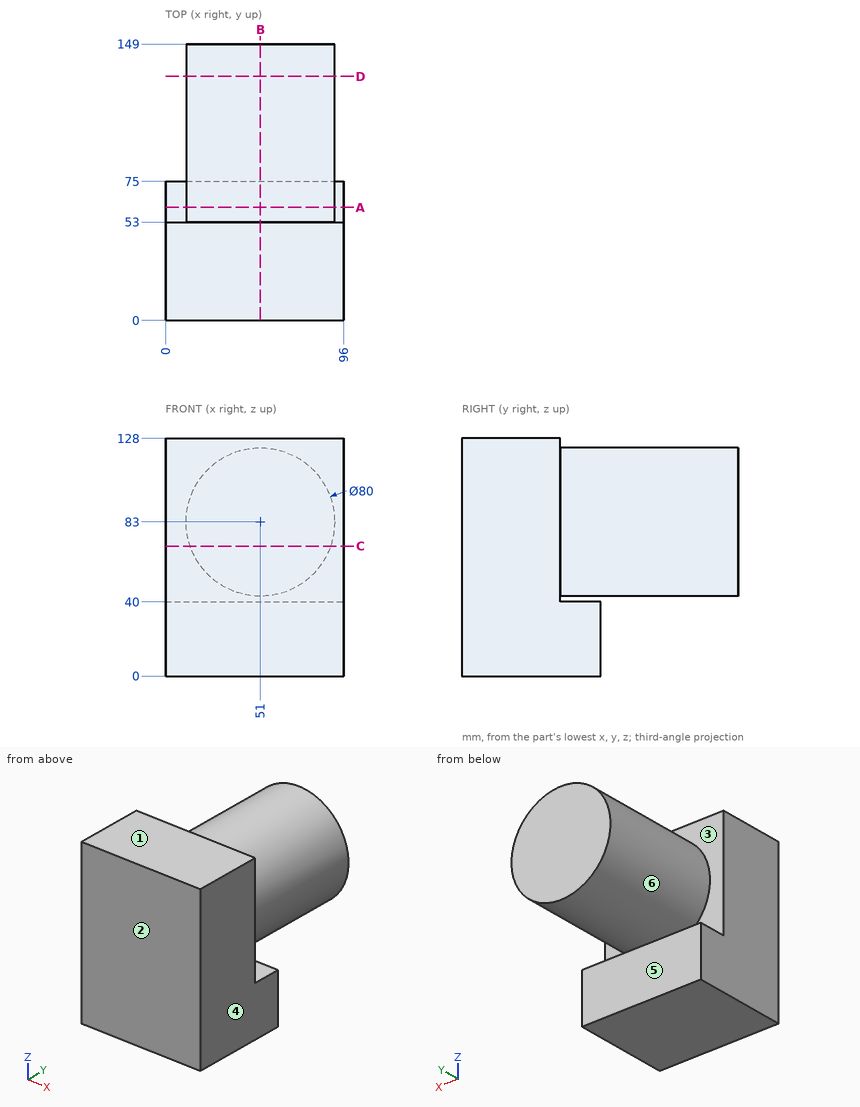
The drawing under review shows one solid part. Ordinate dimensions are in mm from its lowest x, y, z. A direction names the side the tool comes from. Coordinates: 2 decimals unless noted, no trailing zeros. Order: outer loops, then holes, each group sorted by start corner. A loop starts at its lowest first (then second) coordinate and runs counter-clockwise, first axis right, second up. Notation, with made-up numbers: M 86.5,69 L 127.5,69 A10 ccw 127.5,87 Z; hole C 40,-0.75 d5. An arc over 180 degrees is marked long. Use a Markdown table: item, result.
(1) For the marked faces 4, 5 and 6, list the 3-axis set-ups (+Z, -Z, +X, -X, +Y, -Y) from which the entire face can be reached by the end or side of a thin tool; tool diameter is ignored.
Worked answers:
| item | result |
|---|---|
| face 4 | +Z, -Z, +X, +Y, -Y |
| face 5 | -Z, +X, -X, +Y |
| face 6 | +Y |
(2) Add section B-B (x = 51). Give the boundary of the cut face in (y, z), then the cut area to 3 significant figures.
Worked answers:
| item | result |
|---|---|
| outline | M 0,0 L 75,0 L 75,40 L 53,40 L 53,43 L 149,43 L 149,123 L 53,123 L 53,128 L 0,128 Z |
| area | 15,300 mm2 |
(3) Add section A-A (y = 61). Give the boundary of the cut face in (x, z).
Worked answers:
| item | result |
|---|---|
| outline | M 0,0 L 96,0 L 96,40 L 0,40 Z; C 51,83 d80 |
(4) Add section C-C (z = 70). Give the boundary of the cut face in (x, y), then the cut area to 3 significant figures.
Worked answers:
| item | result |
|---|---|
| outline | M 0,0 L 96,0 L 96,53 L 88.83,53 L 88.83,149 L 13.17,149 L 13.17,53 L 0,53 Z |
| area | 12,400 mm2 |
(5) For P1, Ø12, axis at y = 103, z = 112, coming from the -X side; P2, Ø2, axis at y = 60, z = 100.5, coming from the -X side; P3, Ø10, axis at x = 46.5, z = 70, coming from the -Y side; P4, Ø4, axis at y = 77, z = 77, coming from the +X side, all flat-tipped, find the tip position at first contact; note any pin that passes through.
Worked answers:
| item | result |
|---|---|
| P1 | stops at x = 18.27 |
| P2 | stops at x = 14.56 |
| P3 | stops at y = 0 |
| P4 | stops at x = 90.8 |
(6) Add section D-D (y = 131.5). Give the boundary of the cut face in (x, z).
Worked answers:
| item | result |
|---|---|
| outline | C 51,83 d80 |
(7) Wall thickness on probe 1 along Y at (x, z) = (16.5, 111.5); probe 2 along Y at (x, z) = (23, 14); probe 3 along X at (y, z) = (114, 114): over which ranges is each line inside the solid? List them lowest first.
Worked answers:
| item | result |
|---|---|
| probe 1 | y = 0 to 53 |
| probe 2 | y = 0 to 75 |
| probe 3 | x = 25.72 to 76.28 |
(8) Draft analysis for pull direction Z (two halves, no side actions). For the marked faces 1, 2 and 3, state which applies: released by +Z, released by -Z, zero draft, split by the parting line, or undercut.
Worked answers:
| item | result |
|---|---|
| face 1 | released by +Z |
| face 2 | zero draft |
| face 3 | undercut |
